Input: dimensioned drawing with shaded views. Units: mm. Origin: part minimum x, y, z. A direction names the side the tool comes from. Round coordinates to 2 decimals unless told otherwise and drop trailing zeros. Loops run counter-clockwise (first coordinate to the right, second up) from the corner with the lowest first, then second, coordinate; pieces in that order, holes last. Notation, with made-up numbers: (13, -11.75) - (34, -11.75) arc R24 cw to (34, 26.25) - close; hole circle Ø10 at (41.25, -20). An arc over 180 degrees is marked (long way). Answer as a JSON object with one key per item and string values. Group by question number.
Item 1: Section C-C (z = 0.4). Return the cut outline in (x, y).
Item 2: Section A-A (y = 25). Return the cut outline in (x, z), plus the area to 3 significant figures.
Item 3: Line query: line 1 (Y direction, x = 3.1, z = 2.5); line 2 (Z direction, x = 3.15, y = 5); line 3 (Y direction, x = 9.25, z = 2.1). Output: solid intervals per line, ascending.
Item 4: Section B-B (z = 2.5). Return the cut outline in (x, y).
Item 5: Draft query along Y for the marked faces 4, 5, 6 and 7. Return one class per face: released by +Y, released by -Y, zero draft, split by the parting line, or undercut.
Item 6: Reachability of the marked faces 1, 2 and 3 from +Z, -Z, +X, -X, +Y, -Y: full face, straight path, thin tool, end or side. Return the list, or none.
Item 7: First-contact query: pin 1 (2 mm diameter, centred on x = 11.5, z = 2, fed in from -Y); pin 2 (1.5 mm diameter, centred on y = 7.5, z = 3, fed in from +X). Flat tips, straight axial feed; report the tip coordinate or a pass-through.
Item 8: Section D-D (x = 9). Return the cut outline in (y, z).
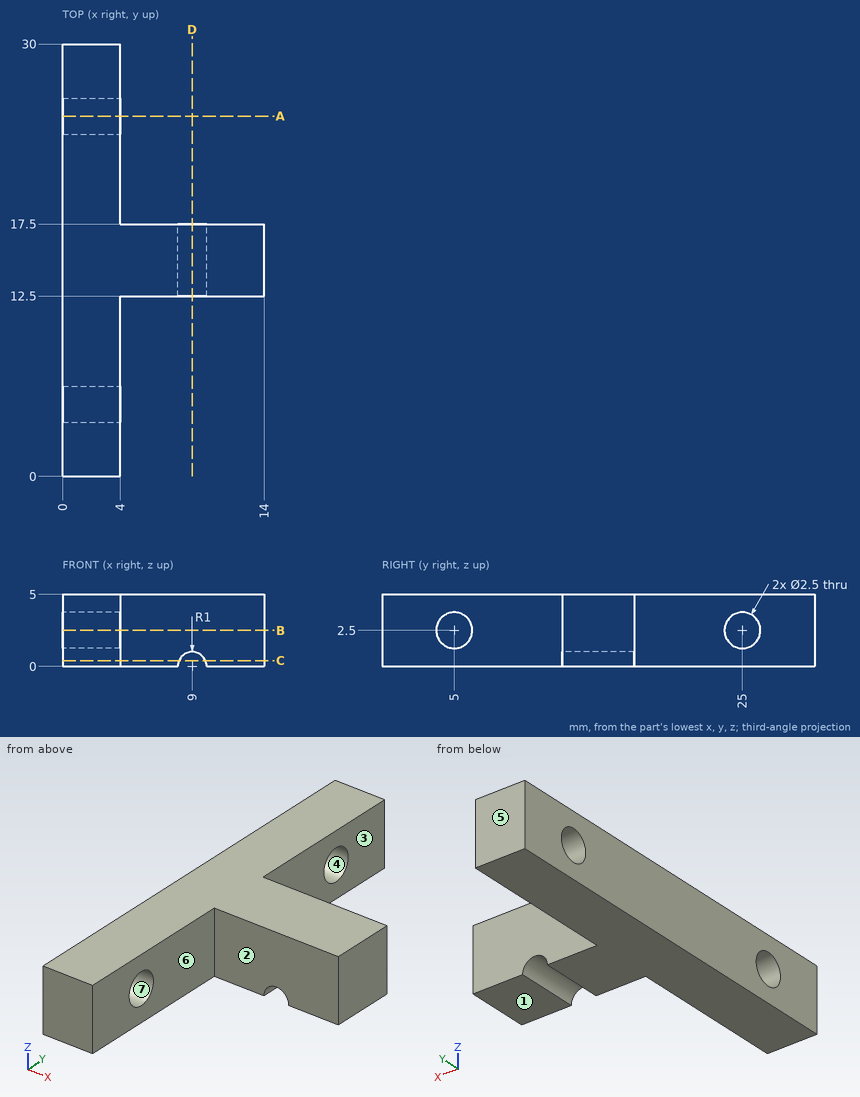
Values:
{
 "1": {"outline": "(0, 0) - (4, 0) - (4, 12.5) - (8.08, 12.5) - (8.08, 17.5) - (4, 17.5) - (4, 30) - (0, 30) - close; (9.92, 12.5) - (14, 12.5) - (14, 17.5) - (9.92, 17.5) - close"},
 "2": {"outline": "(0, 0) - (4, 0) - (4, 1.25) - (0, 1.25) - close; (0, 3.75) - (4, 3.75) - (4, 5) - (0, 5) - close", "area": "10.0 mm^2"},
 "3": {"line 1": "y = 0 to 3.75, 6.25 to 23.75, 26.25 to 30", "line 2": "z = 0 to 1.25, 3.75 to 5", "line 3": "y = 12.5 to 17.5"},
 "4": {"outline": "(0, 0) - (4, 0) - (4, 3.75) - (0, 3.75) - close; (0, 6.25) - (4, 6.25) - (4, 12.5) - (14, 12.5) - (14, 17.5) - (4, 17.5) - (4, 23.75) - (0, 23.75) - close; (0, 26.25) - (4, 26.25) - (4, 30) - (0, 30) - close"},
 "5": {"face 4": "undercut", "face 5": "released by +Y", "face 6": "zero draft", "face 7": "undercut"},
 "6": {"face 1": "-Z, +X, -X, +Y, -Y", "face 2": "+Z, -Z, +X, -Y", "face 3": "+Z, -Z, +X, +Y"},
 "7": {"pin 1": "stops at y = 12.5", "pin 2": "stops at x = 4"},
 "8": {"outline": "(12.5, 1) - (17.5, 1) - (17.5, 5) - (12.5, 5) - close"}
}
